from build123d import *

# Parameters (mm, degrees)
SKETCH_1_R          = 12
EXTRUDE_1_DEPTH     = 4
SKETCH_2_R          = 13
EXTRUDE_2_DEPTH     = 1
SKETCH_3_R          = 7.5
CUT_EXTRUDE_1_DEPTH = 6
FILLET_1_R          = 0.2


with BuildPart() as part:
    # 草图1 → 凸台-拉伸1 (new body)
    with BuildSketch(Plane(origin=(0, 0, 0), x_dir=(0, 0, -1), z_dir=(1, 0, 0))):
        Circle(SKETCH_1_R)
    extrude(amount=EXTRUDE_1_DEPTH)

    # 草图2 → 凸台-拉伸2 (add)
    with BuildSketch(Plane(origin=(4, 0, 0), x_dir=(0, 0, -1), z_dir=(1, 0, 0))):
        Circle(SKETCH_2_R)
    extrude(amount=EXTRUDE_2_DEPTH)

    # 草图3 → 切除-拉伸1 (cut, through all)
    with BuildSketch(Plane.ZY):
        Circle(SKETCH_3_R)
    extrude(amount=-CUT_EXTRUDE_1_DEPTH, mode=Mode.SUBTRACT)

    # 圆角1
    fillet_1_edges = [part.edges().sort_by_distance(p)[0] for p in [
        (0, 0, 12),
        (4, 0, 13),
        (5, 0, 13),
    ]]
    fillet(fillet_1_edges, radius=FILLET_1_R)


solid = part.part
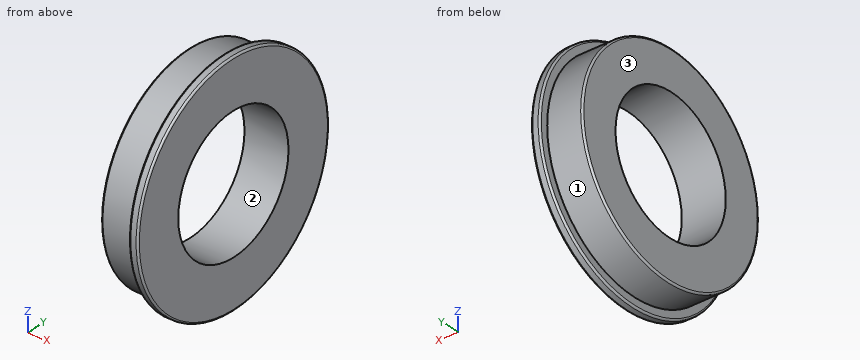
Could you check a few things on this model? Use its own coordinates, in mm. Face numbers are marked on the shaded views. Give positions to 0.01 mm unless a question says otherwise; leave off trailing zeros. Order: outer loops, then holes, each group sorted by start corner. A loop starts at its lowest first (then second) coordinate and runs counter-clockwise, first axis right, second up.
1. Suppose I cut it at C-C (x = 0.9). Write out the boundary of the cut face in (y, z).
Answers below:
outline: circle Ø24 at (0, 0); hole circle Ø15 at (0, 0)
2. Thinking about a two-plate mould opening in Z: for the marked faces 1, 2 and 3, which applies, +Z half, -Z half, draft (parallel to the pull), parting line (faces both ways), or undercut?
Answers below:
face 1: parting line
face 2: undercut
face 3: draft
3. For pin 1 (2 mm diameter, centred on x = 4, z = -2.5, fed in from -Y); pin 2 (1 mm diameter, centred on x = 2, y = 4.5, fed in from -Z); pin 3 (2 mm diameter, centred on x = 2, y = -8, fed in from -Z); pin 4 (10 mm diameter, centred on y = -1.5, z = -2.5, fed in from -X), each with a flat end and sliding along its axis, tell me the tip position at first contact or that it passes through.
Answers below:
pin 1: stops at y = -12.91
pin 2: stops at z = -11.31
pin 3: stops at z = -9.75
pin 4: stops at x = 0
4. I need wall thicknesses on L1, parallel to Y at x = 1.4, z = 0; L2, parallel to Z at x = 4.1, y = 5.25; L3, parallel to Z at x = 0.6, y = -6. Which ranges of each line are inside material? Lowest first, please.
Answers below:
L1: y = -12 to -7.5, 7.5 to 12
L2: z = -11.86 to -5.36, 5.36 to 11.86
L3: z = -10.39 to -4.5, 4.5 to 10.39
5. Suppose I cut it at A-A (z = 0). Write out the boundary of the cut face in (x, y), plus the area to 3 significant figures.
Answers below:
outline: (0, -11.8) arc R0.2 ccw to (0.2, -12) - (4, -12) - (4, -12.8) arc R0.2 ccw to (4.2, -13) - (4.8, -13) arc R0.2 ccw to (5, -12.8) - (5, -7.5) - (0, -7.5) - close; (0, 7.5) - (5, 7.5) - (5, 12.8) arc R0.2 ccw to (4.8, 13) - (4.2, 13) arc R0.2 ccw to (4, 12.8) - (4, 12) - (0.2, 12) arc R0.2 ccw to (0, 11.8) - close
area: 46.9 mm2
